Print and shaded views of the part. All mm, measured from the part's lowest x, y and z. Coordinates: 2 decimals unless noted, no trailing zeros. Order: outer loops, then holes, each group sorted by start corner. A loop starts at its lowest first (then second) coordinate and runs counter-clockwise, first axis right, second up. Notation, with made-up numbers: (81.25, 42) -> (123.25, 42) arc R11 cw to (123.25, 61) -> close; hole circle Ø3 at (24.25, 60). An arc over 180 degrees is marked (long way). Return JSON: item names as keys, results as strings. Group by question number.
1) Cut at D-D (x = 14). Write the cut outline in (y, z), and give its area (3 significant figures).
2) Cut at A-A (x = 26). Write the cut outline in (y, z).
3) Probe line 1 (Y direction, x = 26, z = 1.55); line 2 (X direction, y = 17, z = 6); line 3 (X direction, y = 10, z = 8.75). List the from-to ranges inside material, lowest first.
4) Pull direction X, two halves, no side cores. Call the marked faces 1 and 2: +X half, -X half, draft (parallel to the pull), parting line (faces both ways), or undercut.
5) Cut at C-C (y = 6.5). Write the cut outline in (x, z), and give its area (3 significant figures).
6) Cut at B-B (z = 21.75). Write the cut outline in (x, y).
7) Flat gauge pins, fed straight in: pin 1 (8 mm diameter, centred on x = 17, y = 15.5, fed in from +Z); pin 2 (10 mm diameter, centred on y = 15.5, z = 8, fed in from +X); pin 3 (4 mm diameter, centred on y = 15.5, z = 20.5, fed in from +X). Where does each tip first touch, or does it go through?
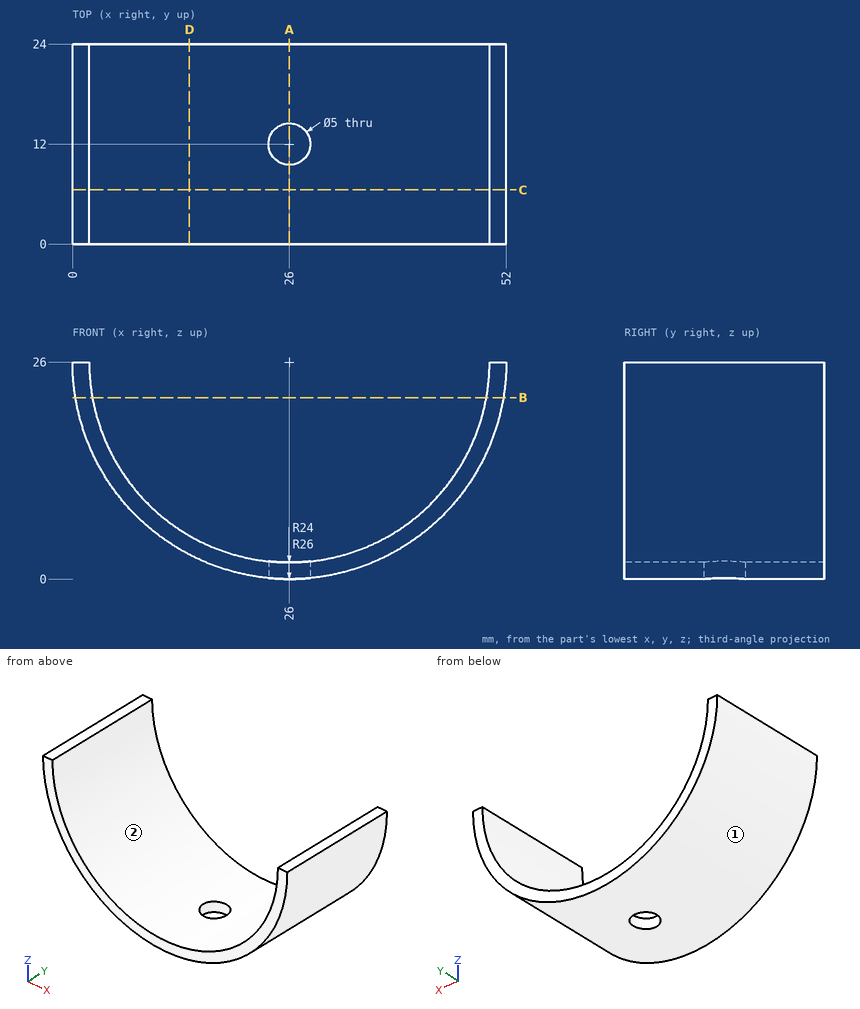
Answers below:
{
 "1": {"outline": "(0, 2.93) -> (24, 2.93) -> (24, 5.22) -> (0, 5.22) -> close", "area": "54.7 mm^2"},
 "2": {"outline": "(0, 0) -> (9.5, 0) -> (9.5, 2) -> (0, 2) -> close; (14.5, 0) -> (24, 0) -> (24, 2) -> (14.5, 2) -> close"},
 "3": {"line 1": "y = 0 to 9.5, 14.5 to 24", "line 2": "x = 9.39 to 12.73, 39.27 to 42.61", "line 3": "x = 6.55 to 9.31, 42.69 to 45.45"},
 "4": {"face 1": "parting line", "face 2": "undercut"},
 "5": {"outline": "(0, 26) arc R26 ccw to (52, 26) -> (50, 26) arc R24 cw to (2, 26) -> close", "area": "157 mm^2"},
 "6": {"outline": "(0.35, 0) -> (2.38, 0) -> (2.38, 24) -> (0.35, 24) -> close; (49.62, 0) -> (51.65, 0) -> (51.65, 24) -> (49.62, 24) -> close"},
 "7": {"pin 1": "stops at z = 5.83", "pin 2": "stops at x = 48.52", "pin 3": "stops at x = 51.76"}
}
